Can you work these out from the model? Positions are in its coordinate system, mm. A direction names the side the tool comes from. Coordinates: 2 decimals unless noted, no trailing zeros. Order: outer loops, then holes, each group sorted by start corner. A loop starts at its lowest first (then second) coordinate and runs counter-clockwise, first axis right, second up. Notation, with made-up numbers: (19.5, 49) -> (45.5, 49) arc R15 cw to (45.5, 62) -> close; hole circle Ø1 at (51, 36). An arc over 180 degrees is marked (long way). Answer in a Markdown table with one row per item.
```python
from build123d import *

# Parameters (mm, degrees)
F1_DEPTH = 0.97852
F2_DEPTH = 2.34214
F3_DEPTH = 3.65164


with BuildPart() as f1:
    # F0 (on Top) → F1 (new body)
    with BuildSketch(Plane.XY):
        with BuildLine():
            Line((0, 5.55195), (5.724427, 5.55195))
            Line((5.724427, 5.55195), (5.724427, 8.900544))
            Line((5.724427, 8.900544), (4.651407, 8.900544))
            ThreePointArc((4.651407, 8.900544), (3.9443, 9.193437), (3.651407, 9.900544))
            Line((3.651407, 9.900544), (3.651407, 18.435233))
            ThreePointArc((3.651407, 18.435233), (3.358514, 19.142339), (2.651407, 19.435233))
            Line((2.651407, 19.435233), (-2.651407, 19.435233))
            ThreePointArc((-2.651407, 19.435233), (-3.358514, 19.142339), (-3.651407, 18.435233))
            Line((-3.651407, 18.435233), (-3.651407, 9.900544))
            ThreePointArc((-3.651407, 9.900544), (-3.9443, 9.193437), (-4.651407, 8.900544))
            Line((-4.651407, 8.900544), (-5.724427, 8.900544))
            Line((-5.724427, 8.900544), (-5.724427, 5.55195))
            Line((-5.724427, 5.55195), (0, 5.55195))
        make_face()
        with BuildLine():
            ThreePointArc((3.651407, 32.429379), (3.358514, 33.136486), (2.651407, 33.429379))
            Line((2.651407, 33.429379), (0, 33.429379))
            Line((0, 33.429379), (-2.651407, 33.429379))
            ThreePointArc((-2.651407, 33.429379), (-3.358514, 33.136486), (-3.651407, 32.429379))
            Line((-3.651407, 32.429379), (-3.651407, 21.738077))
            ThreePointArc((-3.651407, 21.738077), (-3.358514, 21.03097), (-2.651407, 20.738077))
            Line((-2.651407, 20.738077), (2.651407, 20.738077))
            ThreePointArc((2.651407, 20.738077), (3.358514, 21.03097), (3.651407, 21.738077))
            Line((3.651407, 21.738077), (3.651407, 32.429379))
        make_face()
    extrude(amount=F1_DEPTH)

    # F0 (on Top) → F2 (join)
    with BuildSketch(Plane.XY):
        with BuildLine():
            Line((4.651407, 8.900544), (5.724427, 8.900544))
            Line((5.724427, 8.900544), (5.724427, 34.792196))
            Line((5.724427, 34.792196), (0, 34.792196))
            Line((0, 34.792196), (-5.724427, 34.792196))
            Line((-5.724427, 34.792196), (-5.724427, 8.900544))
            Line((-5.724427, 8.900544), (-4.651407, 8.900544))
            ThreePointArc((-4.651407, 8.900544), (-3.9443, 9.193437), (-3.651407, 9.900544))
            Line((-3.651407, 9.900544), (-3.651407, 18.435233))
            ThreePointArc((-3.651407, 18.435233), (-3.358514, 19.142339), (-2.651407, 19.435233))
            Line((-2.651407, 19.435233), (2.651407, 19.435233))
            ThreePointArc((2.651407, 19.435233), (3.358514, 19.142339), (3.651407, 18.435233))
            Line((3.651407, 18.435233), (3.651407, 9.900544))
            ThreePointArc((3.651407, 9.900544), (3.9443, 9.193437), (4.651407, 8.900544))
        make_face()
        with BuildLine():
            Line((0, 33.429379), (2.651407, 33.429379))
            ThreePointArc((2.651407, 33.429379), (3.358514, 33.136486), (3.651407, 32.429379))
            Line((3.651407, 32.429379), (3.651407, 21.738077))
            ThreePointArc((3.651407, 21.738077), (3.358514, 21.03097), (2.651407, 20.738077))
            Line((2.651407, 20.738077), (-2.651407, 20.738077))
            ThreePointArc((-2.651407, 20.738077), (-3.358514, 21.03097), (-3.651407, 21.738077))
            Line((-3.651407, 21.738077), (-3.651407, 32.429379))
            ThreePointArc((-3.651407, 32.429379), (-3.358514, 33.136486), (-2.651407, 33.429379))
            Line((-2.651407, 33.429379), (0, 33.429379))
        make_face(mode=Mode.SUBTRACT)
    extrude(amount=F2_DEPTH)

    # F0 (on Top) → F3 (join)
    with BuildSketch(Plane.XY):
        Polygon((6.567956, 4.76807), (6.567956, 35.9184), (0, 35.9184), (-6.567956, 35.9184), (-6.567956, 4.76807), (0, 4.76807), align=None)
        Polygon((5.724427, 8.900544), (5.724427, 5.55195), (0, 5.55195), (-5.724427, 5.55195), (-5.724427, 8.900544), (-5.724427, 34.792196), (0, 34.792196), (5.724427, 34.792196), align=None, mode=Mode.SUBTRACT)
    extrude(amount=F3_DEPTH)


solid = f1.part
```
(1) Suppose I cut it at D-D (y = 30). Please give me the cut outline in (x, z), and give its area (3 significant figures).
Response values:
| item | result |
|---|---|
| outline | (-6.57, 0) -> (6.57, 0) -> (6.57, 3.65) -> (5.72, 3.65) -> (5.72, 2.34) -> (3.65, 2.34) -> (3.65, 0.98) -> (-3.65, 0.98) -> (-3.65, 2.34) -> (-5.72, 2.34) -> (-5.72, 3.65) -> (-6.57, 3.65) -> close |
| area | 23.0 mm2 |
(2) Suppose I cut it at B-B (x = 1). Please give me the cut outline in (y, z), and give its area (3 significant figures).
Response values:
| item | result |
|---|---|
| outline | (4.77, 0) -> (35.92, 0) -> (35.92, 3.65) -> (34.79, 3.65) -> (34.79, 2.34) -> (33.43, 2.34) -> (33.43, 0.98) -> (20.74, 0.98) -> (20.74, 2.34) -> (19.44, 2.34) -> (19.44, 0.98) -> (5.55, 0.98) -> (5.55, 3.65) -> (4.77, 3.65) -> close |
| area | 39.2 mm2 |
(3) On a 3-axis mill with a long thin cutter (end or side, diameter ignored), from which of +Z, -Z, +X, -X, +Y, -Y can I reach the whole of each face in a straight line? I mean faces 5 (the flat face through (0, 4.768, 2)), 6 (the cylindrical face through (3.37, 21.04, 1.65)). Say none if no direction works.
Response values:
| item | result |
|---|---|
| face 5 | +Z, -Z, +X, -X, -Y |
| face 6 | +Z |
(4) Suppose I cut it at C-C (z = 1.35). Please give me the cut outline in (x, y), and give its area (3 significant figures).
Response values:
| item | result |
|---|---|
| outline | (-6.57, 4.77) -> (6.57, 4.77) -> (6.57, 35.92) -> (-6.57, 35.92) -> close; hole (-5.72, 5.55) -> (5.72, 5.55) -> (5.72, 8.9) -> (4.65, 8.9) arc R1 cw to (3.65, 9.9) -> (3.65, 18.44) arc R1 ccw to (2.65, 19.44) -> (-2.65, 19.44) arc R1 ccw to (-3.65, 18.44) -> (-3.65, 9.9) arc R1 cw to (-4.65, 8.9) -> (-5.72, 8.9) -> close; hole (-3.65, 21.74) arc R1 ccw to (-2.65, 20.74) -> (2.65, 20.74) arc R1 ccw to (3.65, 21.74) -> (3.65, 32.43) arc R1 ccw to (2.65, 33.43) -> (-2.65, 33.43) arc R1 ccw to (-3.65, 32.43) -> close |
| area | 202 mm2 |
(5) Suppose I cut it at A-A (z = 2.7). Please give me the cut outline in (x, y), and give its area (3 significant figures).
Response values:
| item | result |
|---|---|
| outline | (-6.57, 4.77) -> (6.57, 4.77) -> (6.57, 35.92) -> (-6.57, 35.92) -> close; hole (-5.72, 5.55) -> (5.72, 5.55) -> (5.72, 34.79) -> (-5.72, 34.79) -> close |
| area | 74.4 mm2 |
(6) Will these pins go through, and if not, where does the flat tip stop? pin 1 Ø1.5 at (x, y) = (2.5, 11.5) entering from +Z; pin 2 Ø6 at (x, y) = (-3.5, 22) entering from +Z; pin 3 Ø5 at (x, y) = (3, 18) entering from +Z.
Response values:
| item | result |
|---|---|
| pin 1 | z = 0.98 |
| pin 2 | z = 3.65 |
| pin 3 | z = 2.34 |
(7) I need wall thicknesses on line 1 (Y direction, x = 2.75, z = 1.15); line 2 (Y direction, x = -2.75, z = 2.85); line 3 (X direction, y = 30, z = 1.2). Which ranges of each line are inside material? Lowest first, please. Write a range as [from, to].
Response values:
| item | result |
|---|---|
| line 1 | [4.77, 5.55], [19.43, 20.74], [33.42, 35.92] |
| line 2 | [4.77, 5.55], [34.79, 35.92] |
| line 3 | [-6.57, -3.65], [3.65, 6.57] |
(8) We'd pull the mould along X, two halves only. Please class faces 1 (the flat face through (6.568, 20, 2)), 2 (the flat face through (-6, 22, 3.652)), 3 (the flat face through (-6.568, 21, 2)), 4 (the flat face through (-5.724, 20, 3)): +X half, -X half, draft (parallel to the pull), parting line (faces both ways), or undercut.
Response values:
| item | result |
|---|---|
| face 1 | +X half |
| face 2 | draft |
| face 3 | -X half |
| face 4 | undercut |
